For this review, take the finished solid that the model builds, in its own axes (mm). A direction names the side the tool comes from. Give positions to 0.01 mm unless a question says otherwise; leave off trailing zeros. Order: outer loops, then holes, each group sorted by start corner. A loop starts at its lowest first (then second) coordinate and runs counter-clockwise, first axis right, second up. Notation, with made-up numbers: (17.5, 46) - (54.5, 46) arc R25 ccw to (54.5, 72) - close; hole circle Ø1 at (-26, -28.5). An arc over 180 degrees is marked (long way). One line per item, written item: value.
Autodesk Inventor part; units mm, degrees
ref_plane "YZ Plane" through (0, 0, 0) normal (1, 0, 0) x (0, 1, 0)
ref_plane "XZ Plane" through (0, 0, 0) normal (0, 1, 0) x (-1, 0, 0)
ref_plane "XY Plane" through (0, 0, 0) normal (0, 0, 1) x (1, 0, 0)
sketch "Esquisse1" plane through (0, 0, 0) normal (1, 0, 0) x (0, 1, 0)
  line L0 (0, 0) -> (10, 0)
  line L1 (10, 0) -> (10, -65)
  line L2 (10, -65) -> (0, -65)
  line L3 (0, -65) -> (0, 0)
  point P0 (5, -5)
  point P1 (5, -54.2442)
  dimension "d0" = 65
  dimension "d1" = 10
  dimension "d2" = 5
  dimension "d3" = 5
  dimension "d4" = 49.2442
  dimension "d5" = 5
extrude "Extrusion1" add sketch "Esquisse1" along normal blind 3
sketch "Esquisse2" plane through (0, 0, 0) normal (-1, 0, 0) x (0, 0, 1)
  line L0 (-25, 25) -> (15, 25)
  line L1 (15, 25) -> (15, -15)
  line L2 (15, -15) -> (-25, -15)
  line L3 (-25, -15) -> (-25, 25)
  line L4 (-65, 0) -> (0, 0)
  line L5 (0, 0) -> (0, 10)
  line L6 (-50, -10) -> (-80, -10)
  line L7 (-80, -10) -> (-80, 20)
  line L8 (-80, 20) -> (-50, 20)
  line L9 (-50, 20) -> (-50, -10)
  line L10 (-65, 10) -> (-65, 0)
  dimension "d8" = 40
  dimension "d9" = 25
  dimension "d10" = 40
  dimension "d11" = 25
  dimension "d36" = 30
  dimension "d37" = 30
  dimension "d38" = 20
  dimension "d39" = 15
extrude "Extrusion2" add sketch "Esquisse2" against normal blind 3 contours L0 L1 L2 L3
sketch "Esquisse3" plane through (0, 0, 0) normal (-1, 0, 0) x (0, 0, 1)
  line L0 (-65, 10) -> (-25, 10)
  line L1 (-65, 10) -> (-65, 0)
  line L2 (-65, 0) -> (-25, 0)
  circle A0 centre (-60, 5) radius 4
  circle A1 centre (-6.1484, 5) radius 10
  point P0 (0, 0)
  dimension "d14" = 5
  dimension "d15" = 5
  dimension "d16" = 53.8516
  dimension "d17" = 5
  dimension "d18" = 8
  dimension "d19" = 20
extrude "Extrusion3" cut sketch "Esquisse3" against normal blind 3
sketch "Esquisse4" plane through (0, 0, 0) normal (-1, 0, 0) x (0, 0, 1)
  circle A0 centre (-6.1484, 5) radius 10
  circle A1 centre (-6.1484, 5) radius 15
  point P0 (0, 0)
  point P1 (-6.1484, 20)
  point P2 (-19.1388, -2.5)
  point P3 (6.842, -2.5)
  dimension "d22" = 30
  dimension "d25" = 360
hole "Perçage1" at (0, 20, -6.1484) at (0, -2.5, -19.1388) at (0, -2.5, 6.842) direction (1, 0, 0) diameter 3.5 depth 3 tip angle 118
fillet "Congé1" radius 3 2 edges at (1.5, 10, -65) (1.5, 0, -65)
fillet "Congé2" radius 20 4 edges at (1.5, -15, -25) (1.5, 25, -25) (1.5, -15, 15) (1.5, 25, 15)
sketch "Esquisse5" plane through (0, 0, 0) normal (-1, 0, 0) x (0, 0, 1)
  line L0 (-75, 20) -> (-45, 20)
  line L1 (-45, 20) -> (-45, -10)
  line L2 (-45, -10) -> (-75, -10)
  line L3 (-75, -10) -> (-75, 20)
  line L4 (-62, 0) -> (-25, 0)
  line L5 (-65, 7) -> (-65, 3)
  point P0 (0, 0)
  dimension "d40" = 30
  dimension "d41" = 30
  dimension "d42" = 20
  dimension "d43" = 10
extrude "Extrusion4" add sketch "Esquisse5" against normal blind 3
sketch "Esquisse6" plane through (0, 0, 0) normal (-1, 0, 0) x (0, 0, 1)
  line L0 (-75, 20) -> (-45, 20)
  circle A0 centre (-6.1484, 5) radius 10
  point P0 (0, 0)
  point P1 (-60, 5)
  dimension "d46" = 15
  dimension "d47" = 53.8516
hole "Perçage2" at (0, 5, -60) direction (1, 0, 0) diameter 22 depth 3 tip angle 118
fillet "Congé3" radius 15 4 edges at (1.5, -10, -75) (1.5, -10, -45) (1.5, 20, -45) (1.5, 20, -75)
properties part number "barrecodeuse"
(1) Wall thickness on line 1 (Y direction, x = 1.9, z = -6); line 2 (Z direction, x = 1.85, y = 3.5); line 3 (Z direction, x = 1.85, y = 12) (1 decimal): over which ranges is each line inside the solid? List them lowest first. Write a range as from..to.
Answers below:
line 1: y = -15..-5, 15..18.26, 21.74..25
line 2: z = -74.92..-70.9, -49.1..-16.04, 3.74..14.94
line 3: z = -73.3..-68.5, -51.5..-45.9, -24.4..-13.3, 1..13.7
(2) Take a section at A-A (y = 5). Write out the cut boundary in (x, z).
Answers below:
outline: (0, -75) - (3, -75) - (3, -71) - (0, -71) - close; (0, -49) - (3, -49) - (3, -16.15) - (0, -16.15) - close; (0, 3.85) - (3, 3.85) - (3, 15) - (0, 15) - close
(3) Draft analysis for pull direction Y (two halves, no side actions). For faces 1 (the face through (1, 5, -75)), 2 (the face through (1.48, 8, 3.39)), 3 (the face through (1, 10, -35)), state which applies: pulls with the +Y half, pulls with the -Y half, needs draft (parallel to the pull), parting line crosses it, or undercut.
Answers below:
face 1: parting line crosses it
face 2: undercut
face 3: pulls with the +Y half
(4) Take a section at C-C (z = 3). Write out the cut boundary in (x, y), then the cut area to 3 significant figures.
Answers below:
outline: (0, -13.33) - (3, -13.33) - (3, 0.96) - (0, 0.96) - close; (0, 9.04) - (3, 9.04) - (3, 23.33) - (0, 23.33) - close
area: 85.8 mm^2
(5) Machinability: for faces 4 (the face through (1.48, 20.92, -17.74)), 5 (the face through (1.521, 18.265, -6.376)), 6 (the face through (1.479, -10.698, -18.028)), which of the approach directions +Z, -Z, +X, -X, +Y, -Y give a long, thin tool a straight path to every point of the face, cutting with its end or side? Answer none if there is none.
Answers below:
face 4: +X, -X, +Y
face 5: +X, -X
face 6: +X, -X, -Y
(6) For P1, Ø1.5, axis at x = 2, z = -36, coming from the +Y side; P2, Ø3, axis at y = -2.5, z = 6.842, coming from the -X side; P3, Ø1.5, axis at x = 2, z = -34.5, coming from the -Y side; P4, Ø0.9, axis at x = 1.5, z = -59.5, coming from the +Y side, all flat-tipped, find the tip position at first contact; note any pin that passes through.
Answers below:
P1: stops at y = 10
P2: passes through
P3: stops at y = 0
P4: stops at y = 20
(7) Take a section at D-D (z = -69). Write out the cut boundary in (x, y), then the cut area to 3 significant figures.
Answers below:
outline: (0, -7) - (3, -7) - (3, -1.32) - (0, -1.32) - close; (0, 11.32) - (3, 11.32) - (3, 17) - (0, 17) - close
area: 34.1 mm^2
(8) Take a section at B-B (y = -2.5). Write out the cut boundary in (x, z), then the cut area to 3 significant figures.
Answers below:
outline: (0, -72.99) - (3, -72.99) - (3, -68.05) - (0, -68.05) - close; (0, -51.95) - (3, -51.95) - (3, -46.15) - (0, -46.15) - close; (0, -24.18) - (3, -24.18) - (3, -20.89) - (0, -20.89) - close; (0, -17.39) - (3, -17.39) - (3, -12.76) - (0, -12.76) - close; (0, 0.47) - (3, 0.47) - (3, 5.09) - (0, 5.09) - close; (0, 8.59) - (3, 8.59) - (3, 13.54) - (0, 13.54) - close
area: 84.7 mm^2
